Work out the finished part from the listing and answer in its coordinate system (mm). Coordinates: 2 decimals unless noted, no trailing zeros. Write each loop counter-clockwise with the first axis right and the second up, starting at its lowest first coordinate (ties: lowest second). Pieces come first, ordered by that corner, then holes. Notation, with made-up numbers: (-33, 71) - (20, 71) arc R10 cw to (20, 82) - close; hole circle Ø7 at (-7, 30.5). An arc over 180 degrees is marked (long way). Use one line per item in the form item = value. Start each with the question number.
Item 1: Given pin 1 (12 mm diameter, centred on x = 13, y = 4, fed in from +Z); pin 2 (12 mm diameter, centred on x = 25, y = 26, fed in from +Z); pin 3 (5.5 mm diameter, centred on x = 16.5, z = -0.5, fed in from -Y), each flat-ended and moving along its own axis, determine where each tip first touches the part or whether it passes through.
Item 2: A cutting plane is placed at B-B (z = 0). Write down the section's boundary in (x, y).
Item 3: A cutting plane is placed at C-C (x = 45.5). Write down the section's boundary in (y, z), then the cut area to 3 significant figures.
Item 4: Determine the mould class of faces 1 (the cylindrical face through (1.067, -25.268, 77.006)), 2 (the flat face through (1, 3.175, 0)), 3 (the flat face through (76.2, -3, 54)) for opening direction Z: released by +Z, released by -Z, zero draft, split by the parting line, or undercut.
Item 5: A cutting plane is placed at D-D (y = -19). Write down the section's boundary in (x, z), then the cut area to 3 significant figures.
Item 6: Consider probe 1 along Z at (x, y) = (-6.5, 0); probe 2 along Y at (x, z) = (29.5, 0); probe 3 along Z at (x, y) = (33.5, -0.5). Determine where each line is inside the solid, lowest interval first.
Item 7: A cutting plane is placed at A-A (y = -3). Write down the section's boundary in (x, z).
from build123d import *

# Parameters (mm, degrees)
BOSS_EXTRUDE1_DEPTH = 76.2


with BuildPart() as part:
    # Sketch1 → Boss-Extrude1 (new, symmetric)
    with BuildSketch(Plane(origin=(0, 0, 0), x_dir=(0, 0, -1), z_dir=(1, 0, 0))):
        with BuildLine():
            ThreePointArc((-4.852064404, 24.93225764), (23.991364551, 8.341128638), (11.661357948, -22.5648561))
            ThreePointArc((11.661357948, -22.5648561), (-78.193446496, -24.733850104), (-135.351657349, 44.631338202))
            ThreePointArc((-135.351657349, 44.631338202), (-71.80288322, 23.513113441), (-4.852064404, 24.93225764))
        make_face()
        with BuildLine():
            Line((-5.4991, 3.175279388), (5.4991, 3.175279388))
            ThreePointArc((5.4991, 3.175279388), (0, -6.35), (-5.4991, 3.175279388))
        make_face(mode=Mode.SUBTRACT)
    extrude(amount=BOSS_EXTRUDE1_DEPTH, both=True)


solid = part.part
Answer:
q1.pin_1 = 119.79
q1.pin_2 = 131.43
q1.pin_3 = -28.5
q2.outline = (-76.2, -27.7) - (76.2, -27.7) - (76.2, -6.35) - (-76.2, -6.35) - close; (-76.2, 3.18) - (76.2, 3.18) - (76.2, 25.4) - (-76.2, 25.4) - close
q3.outline = (-22.56, -11.66) arc R25.4 ccw to (24.93, 4.85) arc R196.75 cw to (44.63, 135.35) arc R102.71 ccw to start; hole (3.18, -5.5) - (3.18, 5.5) arc R6.35 ccw (long way) to start
q3.area = 7,090 mm²
q4.face_1 = split by the parting line
q4.face_2 = undercut
q4.face_3 = zero draft
q5.outline = (-76.2, -16.86) - (76.2, -16.86) - (76.2, 88.99) - (-76.2, 88.99) - close
q5.area = 16,100 mm²
q6.probe_1 = -25.4 to -6.35, 6.35 to 111.87
q6.probe_2 = -27.7 to -6.35, 3.18 to 25.4
q6.probe_3 = -25.4 to -6.33, 6.33 to 111.41
q7.outline = (-76.2, -25.22) - (76.2, -25.22) - (76.2, -5.6) - (-76.2, -5.6) - close; (-76.2, 5.6) - (76.2, 5.6) - (76.2, 109.06) - (-76.2, 109.06) - close
